Autodesk Inventor part; units mm, degrees
ref_plane "YZ Plane" through (0, 0, 0) normal (1, 0, 0) x (0, 1, 0)
ref_plane "XZ Plane" through (0, 0, 0) normal (0, 1, 0) x (-1, 0, 0)
ref_plane "XY Plane" through (0, 0, 0) normal (0, 0, 1) x (1, 0, 0)
sketch3d "3D Sketch1"
sketch "Sketch8" plane through (0, 0, 0) normal (0, 1, 0) x (-1, 0, 0)
  arc A0 (-533.9727, 129.2939) -> (-533.9727, 72.7061) centre (-524, 101) ccw
  arc A1 (-533.9727, 129.2939) -> (-540.6211, 148.1565) centre (-537.2969, 138.7252) ccw
  arc A2 (-540.6211, 148.1565) -> (-540.6211, 53.8435) centre (-524, 101) ccw
  arc A3 (-540.6211, 53.8435) -> (-533.9727, 72.7061) centre (-537.2969, 63.2748) ccw
  circle A4 centre (-537.2969, 63.2748) radius 3
  circle A5 centre (-556.6482, 77.8001) radius 2.9994
  circle A6 centre (-564, 101) radius 3
  circle A7 centre (-556.6482, 124.1094) radius 2.9994
  circle A8 centre (-537.2969, 138.7252) radius 3
  line L0 (-531, 98.5) -> (-531, 115.5)
  line L1 (-451.3425, 101.8066) -> (-466.8633, 88.0104)
  arc A9 (-451.3425, 101.8066) -> (-450, 104.7963) centre (-454, 104.7963) ccw
  line L2 (-450, 109.2037) -> (-450, 104.7963)
  arc A10 (-450, 109.2037) -> (-451.3425, 112.1934) centre (-454, 109.2037) ccw
  line L3 (-466.8633, 125.9896) -> (-451.3425, 112.1934)
  arc A11 (-466.8633, 125.9896) -> (-469.5208, 127) centre (-469.5208, 123) ccw
  line L4 (-505.0775, 127) -> (-469.5208, 127)
  arc A12 (-505.0775, 127) -> (-508.201, 125.4988) centre (-505.0775, 123) ccw
  line L5 (-511.799, 121.0012) -> (-508.201, 125.4988)
  arc A13 (-514.9225, 119.5) -> (-511.799, 121.0012) centre (-514.9225, 123.5) ccw
  line L6 (-527, 119.5) -> (-514.9225, 119.5)
  arc A14 (-527, 119.5) -> (-531, 115.5) centre (-527, 115.5) ccw
  arc A15 (-531, 98.5) -> (-527, 94.5) centre (-527, 98.5) ccw
  line L7 (-514.9225, 94.5) -> (-527, 94.5)
  arc A16 (-511.799, 92.9988) -> (-514.9225, 94.5) centre (-514.9225, 90.5) ccw
  line L8 (-508.201, 88.5012) -> (-511.799, 92.9988)
  arc A17 (-508.201, 88.5012) -> (-505.0775, 87) centre (-505.0775, 91) ccw
  line L9 (-469.5208, 87) -> (-505.0775, 87)
  line L10 (-478, 91.45) -> (-470, 91.45)
  arc A18 (-470, 91.45) -> (-470, 94.55) centre (-470, 93) ccw
  line L11 (-470, 94.55) -> (-478, 94.55)
  arc A19 (-478, 94.55) -> (-478, 91.45) centre (-478, 93) ccw
  arc A20 (-495, 91.45) -> (-495, 94.55) centre (-495, 93) ccw
  line L12 (-503, 91.45) -> (-495, 91.45)
  arc A21 (-503, 94.55) -> (-503, 91.45) centre (-503, 93) ccw
  line L13 (-495, 94.55) -> (-503, 94.55)
  line L14 (-455, 105.5) -> (-469, 105.5)
  arc A22 (-455, 105.5) -> (-455, 108.5) centre (-455, 107) ccw
  line L15 (-469, 108.5) -> (-455, 108.5)
  arc A23 (-469, 108.5) -> (-469, 105.5) centre (-469, 107) ccw
  arc A24 (-482, 105.45) -> (-482, 108.55) centre (-482, 107) ccw
  line L16 (-490, 105.45) -> (-482, 105.45)
  arc A25 (-490, 108.55) -> (-490, 105.45) centre (-490, 107) ccw
  line L17 (-482, 108.55) -> (-490, 108.55)
  line L18 (-501, 109) -> (-501, 105)
  line L19 (-501, 105) -> (-511, 105)
  line L20 (-511, 105) -> (-511, 109)
  line L21 (-511, 109) -> (-501, 109)
  circle A26 centre (-525.75, 100) radius 1.55
  circle A27 centre (-525.75, 114) radius 1.55
  arc A28 (-503, 122.55) -> (-503, 119.45) centre (-503, 121) ccw
  line L22 (-503, 122.55) -> (-495, 122.55)
  arc A29 (-495, 119.45) -> (-495, 122.55) centre (-495, 121) ccw
  line L23 (-495, 119.45) -> (-503, 119.45)
  arc A30 (-478, 122.55) -> (-478, 119.45) centre (-478, 121) ccw
  line L24 (-478, 122.55) -> (-470, 122.55)
  arc A31 (-470, 119.45) -> (-470, 122.55) centre (-470, 121) ccw
  line L25 (-470, 119.45) -> (-478, 119.45)
  arc A32 (-469.5208, 87) -> (-466.8633, 88.0104) centre (-469.5208, 91) ccw
  line L26 (-487, 7.43) -> (-478.1, 7.43)
  line L27 (-495.9, 7.43) -> (-487, 7.43)
  arc A33 (-495.9, 7.43) -> (-499.5, 3.83) centre (-495.9, 3.83) ccw
  line L28 (-499.5, -0.5942) -> (-499.5, 3.83)
  arc A34 (-499.5, -0.5942) -> (-498.1907, -3.5539) centre (-495.5, -0.5942) ccw
  line L29 (-490, -11) -> (-498.1907, -3.5539)
  line L30 (-484, -11) -> (-490, -11)
  line L31 (-475.8093, -3.5539) -> (-484, -11)
  arc A35 (-475.8093, -3.5539) -> (-474.5, -0.5942) centre (-478.5, -0.5942) ccw
  line L32 (-474.5, 3.83) -> (-474.5, -0.5942)
  arc A36 (-474.5, 3.83) -> (-478.1, 7.43) centre (-478.1, 3.83) ccw
  arc A37 (-478.45, 4) -> (-481.55, 4) centre (-480, 4) ccw
  line L33 (-481.55, 4) -> (-481.55, -1)
  arc A38 (-481.55, -1) -> (-478.45, -1) centre (-480, -1) ccw
  line L34 (-478.45, -1) -> (-478.45, 4)
  line L35 (-492.45, 4) -> (-492.45, -1)
  arc A39 (-492.45, 4) -> (-495.55, 4) centre (-494, 4) ccw
  line L36 (-495.55, -1) -> (-495.55, 4)
  arc A40 (-495.55, -1) -> (-492.45, -1) centre (-494, -1) ccw
  arc A41 (-494.09, 79.2321) -> (-479.91, 79.2321) centre (-487, 84) ccw
  arc A42 (-494.09, 79.2321) -> (-497.4092, 81) centre (-497.4092, 77) ccw
  line L37 (-497.4092, 81) -> (-503, 81)
  arc A43 (-503, 81) -> (-507, 77) centre (-503, 77) ccw
  line L38 (-507, 77) -> (-507, 50.7937)
  arc A44 (-511.1379, 43.7877) -> (-507, 50.7937) centre (-515, 50.7937) ccw
  arc A45 (-511.1379, 43.7877) -> (-462.8621, 43.7877) centre (-487, 0) ccw
  arc A46 (-467, 50.7937) -> (-462.8621, 43.7877) centre (-459, 50.7937) ccw
  line L39 (-467, 50.7937) -> (-467, 77)
  arc A47 (-467, 77) -> (-471, 81) centre (-471, 77) ccw
  line L40 (-471, 81) -> (-476.5908, 81)
  arc A48 (-476.5908, 81) -> (-479.91, 79.2321) centre (-476.5908, 77) ccw
  circle A49 centre (-473, 75) radius 1.25
  circle A50 centre (-501, 75) radius 1.25
  circle A51 centre (-487, 63) radius 1.25
  circle A52 centre (-470.7, 62.6926) radius 1.25
  circle A53 centre (-473, 50) radius 1.25
  circle A54 centre (-501, 50) radius 1.25
  circle A55 centre (-470.7, 37.4926) radius 1.25
  arc A56 (-485, 53) -> (-489, 53) centre (-487, 53) ccw
  line L41 (-485, 37) -> (-485, 53)
  line L42 (-489, 53) -> (-489, 37)
  arc A57 (-489, 37) -> (-485, 37) centre (-487, 37) ccw
  arc A58 (-513.2873, 34.029) -> (-460.7127, 34.0291) centre (-487, 0) ccw
  arc A59 (-509.6193, 29.2808) -> (-464.3807, 29.2808) centre (-487, 0) ccw
  arc A60 (-460.7127, 34.0291) -> (-464.3807, 29.2808) centre (-462.5467, 31.6549) ccw
  arc A61 (-509.6193, 29.2808) -> (-513.2873, 34.029) centre (-511.4533, 31.6549) ccw
  arc A62 (-496, 32) -> (-500, 28) centre (-496, 28) ccw
  line L43 (-496, 32) -> (-478, 32)
  arc A63 (-474, 28) -> (-478, 32) centre (-478, 28) ccw
  line L44 (-474, 28) -> (-474, 22)
  arc A64 (-474, 22) -> (-470, 18) centre (-470, 22) ccw
  line L45 (-470, 18) -> (-465.0911, 18)
  arc A65 (-461.7205, 16.1538) -> (-465.0911, 18) centre (-465.0911, 14) ccw
  arc A66 (-512.2795, 16.1538) -> (-461.7205, 16.1538) centre (-487, 0) ccw
  arc A67 (-508.9089, 18) -> (-512.2795, 16.1538) centre (-508.9089, 14) ccw
  line L46 (-508.9089, 18) -> (-504, 18)
  arc A68 (-504, 18) -> (-500, 22) centre (-504, 22) ccw
  line L47 (-500, 22) -> (-500, 28)
  point P0 (0, 0)
extrude "Extrusion1" add sketch "Sketch8" along normal blind 3 contours L26 A36 L32 A35 L31 L30 L29 A34 L28 A33 L27
properties part number "pulsador_punta"
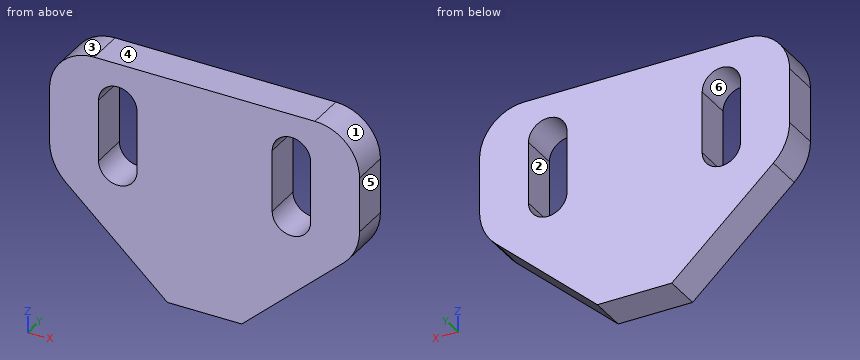
Verification items for the finished model (mm, model axes). Face numbers are marked on the shaded views. A direction names the side the tool comes from. Coordinates: 2 decimals unless noted, no trailing zeros. Order: outer loops, then holes, each group sorted by start corner. A loop starts at its lowest first (then second) coordinate and runs counter-clockwise, first axis right, second up. Notation, with made-up numbers: (83.5, 16) -> (117.5, 16) arc R15 ccw to (117.5, 28) -> close; hole circle Ø9 at (48, 89.5). An arc over 180 degrees is marked (long way). Put each result on its own line as item: value. Start each with the question number.
1) Cross-section at B-B (y = 0.9). Enter the section's corners in (x, z), plus the area to 3 significant figures.
2) Cross-section at C-C (x = 494). Enter the section's corners in (y, z), plus the area to 3 significant figures.
3) Release check for a two-part mould opening along X. For the marked faces 1, 2, 3 and 4 record: pulls with the +X half, pulls with the -X half, needs draft (parallel to the pull), parting line crosses it, or undercut.
4) Cross-section at A-A (z = 1). Enter the section's corners in (x, y), plus the area to 3 significant figures.
5) Material ranges on L1, parallel to X at y = 0.3, z = 3.75; L2, parallel to X at y = 1.7, z = 4.25; L3, parallel to Z at x = 480.5, y = 1.1, recorded low to high.
6) Go/stop test with a flat-tipped pin: pin 1 (1 mm diameter, centred on y = 0.5, z = -4, fed in from -X). Record where the tip stops, or that it passes through.
7) Cross-section at D-D (z = 4.75). Enter the section's corners in (x, y).
8) Tool access check on the marked faces 5 and 6. Record the directions out of +Z, -Z, +X, -X, +Y, -Y that give a thin tool (end or side, any length) a straight path to the whole face; none if there is none.
Geometry check:
1. outline: (474.5, -0.59) arc R4 ccw to (475.81, -3.55) -> (484, -11) -> (490, -11) -> (498.19, -3.55) arc R4 ccw to (499.5, -0.59) -> (499.5, 3.83) arc R3.6 ccw to (495.9, 7.43) -> (478.1, 7.43) arc R3.6 ccw to (474.5, 3.83) -> close; hole (478.45, -1) arc R1.55 ccw to (481.55, -1) -> (481.55, 4) arc R1.55 ccw to (478.45, 4) -> close; hole (492.45, -1) arc R1.55 ccw to (495.55, -1) -> (495.55, 4) arc R1.55 ccw to (492.45, 4) -> close
1. area: 326 mm^2
2. outline: (0, -7.36) -> (3, -7.36) -> (3, -2.55) -> (0, -2.55) -> close; (0, 5.55) -> (3, 5.55) -> (3, 7.43) -> (0, 7.43) -> close
2. area: 20.1 mm^2
3. face 1: pulls with the +X half
3. face 2: undercut
3. face 3: pulls with the -X half
3. face 4: needs draft
4. outline: (474.5, 0) -> (478.45, 0) -> (478.45, 3) -> (474.5, 3) -> close; (481.55, 0) -> (492.45, 0) -> (492.45, 3) -> (481.55, 3) -> close; (495.55, 0) -> (499.5, 0) -> (499.5, 3) -> (495.55, 3) -> close
4. area: 56.4 mm^2
5. L1: x = 474.5 to 478.45, 481.55 to 492.45, 495.55 to 499.5
5. L2: x = 474.52 to 478.47, 481.53 to 492.47, 495.53 to 499.48
5. L3: z = -7.82 to -2.47, 5.47 to 7.43
6. pin 1: stops at x = 475.75
7. outline: (474.62, 0) -> (478.64, 0) -> (478.64, 3) -> (474.62, 3) -> close; (481.36, 0) -> (492.64, 0) -> (492.64, 3) -> (481.36, 3) -> close; (495.36, 0) -> (499.38, 0) -> (499.38, 3) -> (495.36, 3) -> close
8. face 5: +Z, -Z, +X, +Y, -Y
8. face 6: +Y, -Y
